from build123d import *

# Parameters (mm, degrees)
SKETCH_R          = 12.5
PAD_DEPTH         = 68.5
SKETCH001_W       = 3.5
SKETCH001_H       = 25
POCKET_DEPTH      = 68.501
POCKET_DEPTH_BACK = -68.501
SKETCH002_W       = 3.5
SKETCH002_H       = 30
POCKET001_DEPTH   = 15


with BuildPart() as part:
    # Sketch → Pad (new body, symmetric)
    with BuildSketch(Plane.XZ):
        Circle(SKETCH_R)
    extrude(amount=PAD_DEPTH, both=True)

    # Sketch001 → Pocket (cut, two sides)
    with BuildSketch(Plane.XZ) as pocket_sk:
        with Locations((0, -9.5)):
            Rectangle(SKETCH001_W, SKETCH001_H)
    extrude(amount=-POCKET_DEPTH, mode=Mode.SUBTRACT)
    extrude(pocket_sk.sketch, amount=-POCKET_DEPTH_BACK, mode=Mode.SUBTRACT)

    # Sketch002 → Pocket001 (cut)
    with BuildSketch(Plane.XZ.offset(68.5)):
        Rectangle(SKETCH002_W, SKETCH002_H)
    pocket001 = extrude(amount=-POCKET001_DEPTH, mode=Mode.SUBTRACT)

    # Mirrored: Pocket001 across XZ
    add(pocket001.mirror(Plane.XZ), mode=Mode.SUBTRACT)


solid = part.part
Design review of the part built by this model. Coordinates are the model's own, in mm. A direction names the side the tool comes from. Coordinates: 2 decimals unless noted, no trailing zeros. Order: outer loops, then holes, each group sorted by start corner. A loop starts at its lowest first (then second) coordinate and runs counter-clockwise, first axis right, second up.
Item 1: For line 1 (X direction, y = -59, z = -1.75); line 2 (X direction, y = 45, z = -2); line 3 (Z direction, x = -0.75, y = -9), list the stretches that pass through material, from the lowest coordinate up.
Item 2: Take a section at C-C, the plane z = 5.5. Write out the cut boundary in (x, y).
Item 3: For pin 1 Ø10 at (x, y) = (9.5, -17.5) entering from -Z; pin 2 Ø1.5 at (y, z) = (16.5, 1) entering from +X; pin 3 Ø3 at (y, z) = (-39.5, -8) entering from -X, all flat-tipped, find the tip position at first contact; note any pin that passes through.
Item 4: The part is to be moulded in two halves that separate along X. For faces 1 (the flat face through (1.75, -1, -3)), 2 (the flat face through (6, -68.5, 0)), 3 (the cylindrical face through (0.53, -0.96, 12.49)), say which applies: pulls with the +X half, pulls with the -X half, needs draft (parallel to the pull), parting line crosses it, or undercut.
Item 5: Take a section at B-B, the plane x = 0. Write out the cut boundary in (y, z).
Item 6: For faces 4 (the flat face through (-6, -68.5, 0)), 5 (the flat face through (0, -53.5, 8)), 6 (the flat face through (0, 53.5, 8)), 7 (the flat face through (0, -1, 3)), 8 (the flat face through (6, 68.5, 0)), list the 3-axis set-ups (+Z, -Z, +X, -X, +Y, -Y) from which the entire face can be reached by the end or side of a thin tool; tool diameter is ignored.
Item 7: Take a section at D-D, the plane y = -47. Write out the cut boundary in (x, z).
Item 8: Take a section at A-A, the plane z = 0. Write out the cut boundary in (x, y), then the cut area to 3 significant figures.
The answers:
1. line 1: x = -12.38 to -1.75, 1.75 to 12.38
1. line 2: x = -12.34 to -1.75, 1.75 to 12.34
1. line 3: z = 3 to 12.48
2. outline: (-11.22, -68.5) - (-1.75, -68.5) - (-1.75, -53.5) - (1.75, -53.5) - (1.75, -68.5) - (11.22, -68.5) - (11.22, 68.5) - (1.75, 68.5) - (1.75, 53.5) - (-1.75, 53.5) - (-1.75, 68.5) - (-11.22, 68.5) - close
3. pin 1: stops at z = -11.66
3. pin 2: stops at x = 12.5
3. pin 3: stops at x = -10.68
4. face 1: undercut
4. face 2: needs draft
4. face 3: parting line crosses it
5. outline: (-53.5, 3) - (53.5, 3) - (53.5, 12.5) - (-53.5, 12.5) - close
6. face 4: +Z, -Z, +X, -X, -Y
6. face 5: +Z, -Z, -Y
6. face 6: +Z, -Z, +Y
6. face 7: -Z, +Y, -Y
6. face 8: +Z, -Z, +X, -X, +Y
7. outline: (-1.75, -12.38) - (-1.75, 3) - (1.75, 3) - (1.75, -12.38) arc R12.5 ccw (long way) to start
8. outline: (-12.5, -68.5) - (-1.75, -68.5) - (-1.75, 68.5) - (-12.5, 68.5) - close; (1.75, -68.5) - (12.5, -68.5) - (12.5, 68.5) - (1.75, 68.5) - close
8. area: 2,950 mm2
